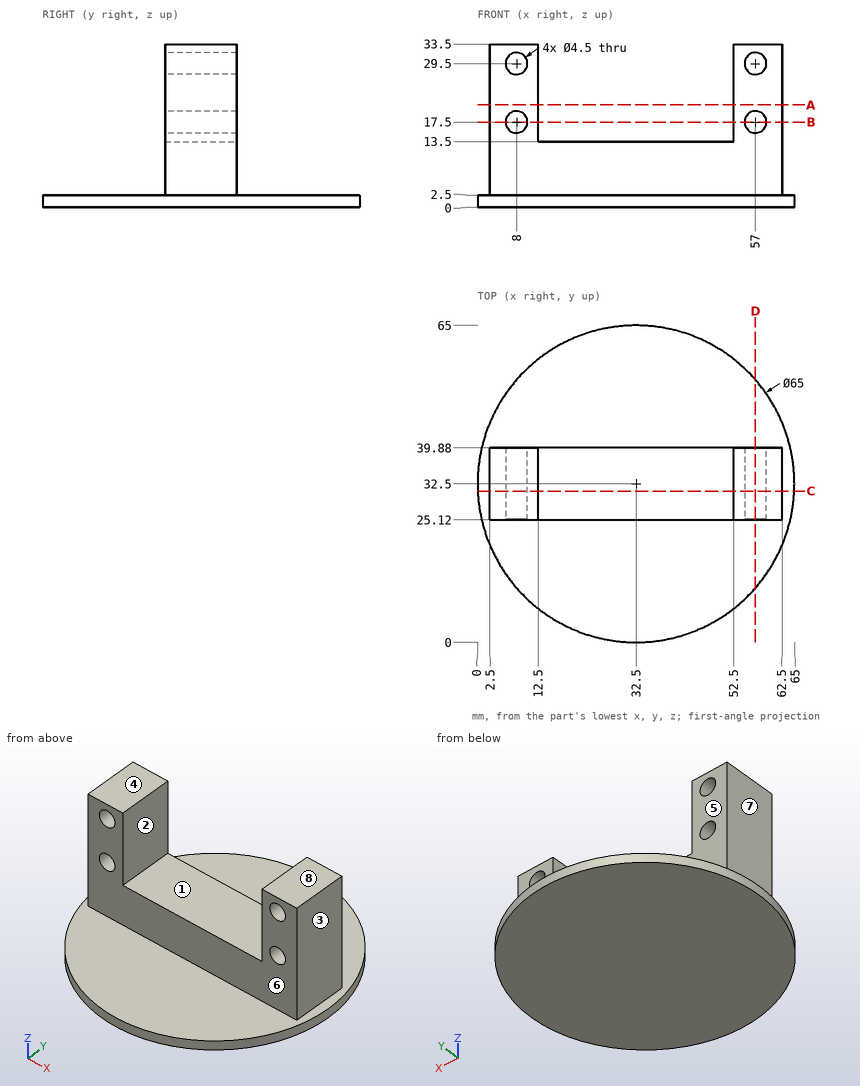
Verification items for this drawing (mm, ordinates from the low corner). A direction names the side the tool comes from. Coordinates: 2 decimals unless noted, no trailing zeros. Order: outer loops, then holes, each group sorted by start corner. A loop starts at its lowest first (then second) coordinate and runs counter-clockwise, first axis right, second up. Notation, with made-up numbers: (6, 26.5) - (47, 26.5) arc R21 ccw to (47, 39.5) - close; hole circle Ø5 at (-28.75, -9). An arc over 180 degrees is marked (long way). Use one line per item in the form item = value.
1. Section check D-D (x = 57). Record the boundary of the cut face in (y, z).
Here are the results:
outline = (11.15, 0) - (53.85, 0) - (53.85, 2.5) - (39.88, 2.5) - (39.88, 15.25) - (25.12, 15.25) - (25.12, 2.5) - (11.15, 2.5) - close; (25.12, 19.75) - (39.88, 19.75) - (39.88, 27.25) - (25.12, 27.25) - close; (25.12, 31.75) - (39.88, 31.75) - (39.88, 33.5) - (25.12, 33.5) - close
2. Access from +Z, -Z, +X, -X, +Y, -Y to the whole of each face (thin tool, end or side, straight path). Record for the marked faces 5, 6, 7 and 8.
Here are the results:
face_5 = +Z, +X, -X, +Y
face_6 = +Z, +X, -X, -Y
face_7 = +Z, -X, +Y, -Y
face_8 = +Z, +X, -X, +Y, -Y
3. Draft check along X on the marked faces 1, 2, 3 and 4. Enter one of: pulls with the +X half, pulls with the -X half, needs draft (parallel to the pull), parting line crosses it, or undercut.
Here are the results:
face_1 = undercut
face_2 = undercut
face_3 = pulls with the +X half
face_4 = needs draft
4. Gauge pin test, flat ends, axial feed: pin 1 (5 mm diameter, centred on x = 57.5, z = 19.5, fed in from -Y); pin 2 (4.5 mm diameter, centred on x = 36.5, y = 33, fed in from +Z); pin 3 (6 mm diameter, centred on x = 57, z = 17.5, fed in from +Y). Record the tip position at first contact, or that the pin passes through.
Here are the results:
pin_1 = 25.12
pin_2 = 13.5
pin_3 = 39.88
5. Section check A-A (z = 21). Record the boundary of the cut face in (x, y).
Here are the results:
outline = (2.5, 25.12) - (12.5, 25.12) - (12.5, 39.88) - (2.5, 39.88) - close; (52.5, 25.12) - (62.5, 25.12) - (62.5, 39.88) - (52.5, 39.88) - close
6. Section check B-B (z = 17.5). Record the boundary of the cut face in (x, y).
Here are the results:
outline = (2.5, 25.12) - (5.75, 25.12) - (5.75, 39.88) - (2.5, 39.88) - close; (10.25, 25.12) - (12.5, 25.12) - (12.5, 39.88) - (10.25, 39.88) - close; (52.5, 25.12) - (54.75, 25.12) - (54.75, 39.88) - (52.5, 39.88) - close; (59.25, 25.12) - (62.5, 25.12) - (62.5, 39.88) - (59.25, 39.88) - close
7. Scan lines: line 1 (Z direction, x = 57, y = 35); line 2 (X direction, y = 31, z = 20.5); line 3 (Z direction, x = 16, y = 9). Record each from-to range of solid material in increasing order.
Here are the results:
line_1 = 0 to 15.25, 19.75 to 27.25, 31.75 to 33.5
line_2 = 2.5 to 12.5, 52.5 to 62.5
line_3 = 0 to 2.5
8. Section check C-C (y = 31). Record the boundary of the cut face in (x, z).
Here are the results:
outline = (0.03, 0) - (64.97, 0) - (64.97, 2.5) - (62.5, 2.5) - (62.5, 33.5) - (52.5, 33.5) - (52.5, 13.5) - (12.5, 13.5) - (12.5, 33.5) - (2.5, 33.5) - (2.5, 2.5) - (0.03, 2.5) - close; hole circle Ø4.5 at (8, 17.5); hole circle Ø4.5 at (8, 29.5); hole circle Ø4.5 at (57, 17.5); hole circle Ø4.5 at (57, 29.5)
